Autodesk Inventor part; units mm, degrees
ref_plane "YZ Plane" through (0, 0, 0) normal (1, 0, 0) x (0, 1, 0)
ref_plane "XZ Plane" through (0, 0, 0) normal (0, 1, 0) x (-1, 0, 0)
ref_plane "XY Plane" through (0, 0, 0) normal (0, 0, 1) x (1, 0, 0)
sketch "スケッチ1" plane through (0, 0, 0) normal (0, 0, 1) x (1, 0, 0)
  line L0 (-81.3, 0) -> (81.3, 0)
  line L1 (81.3, 0) -> (81.3, 14.5)
  line L2 (81.3, 14.5) -> (-81.3, 14.5)
  line L3 (-81.3, 14.5) -> (-81.3, 0)
  line L4 (-99, 14.5) -> (99, 14.5)
  line L5 (99, 14.5) -> (99, 54.5)
  line L6 (99, 54.5) -> (-99, 54.5)
  line L7 (-99, 54.5) -> (-99, 14.5)
  point P0 (0, 0)
  point P1 (0, 0)
  point P2 (0, 14.5)
  point P3 (-81.3, 14.5)
  point P4 (81.3, 14.5)
  dimension "d0" = 162.6
  dimension "d1" = 14.5
  dimension "d2" = 198
  dimension "d3" = 40
extrude "押し出し1" add sketch "スケッチ1" along normal blind 2.5
properties part number "wall" material "木材 (カエデ材)"
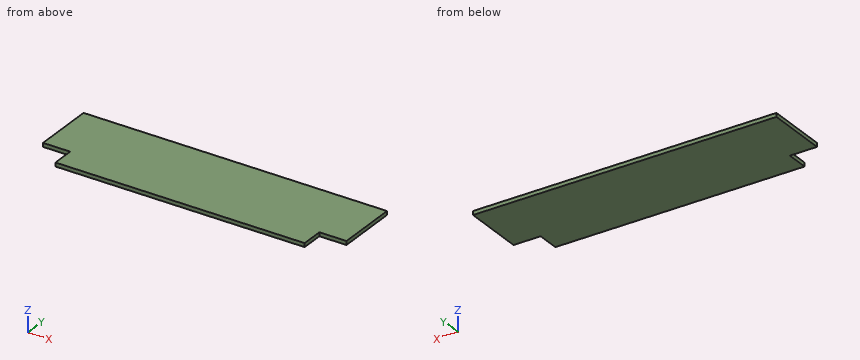
Can you work these out from the model? Positions are in its coordinate system, mm. Coordinates: 2 decimals unless noted, no trailing zeros. Write each loop counter-clockwise with the first axis right and the second up, starting at its lowest first coordinate (ties: lowest second). Pieces come first, ordered by that corner, then holes. Notation, with made-up numbers: (86, 0) -> (100, 0) arc R13 cw to (100, 21) -> close; hole circle Ø1 at (-35.5, 66). An arc over 180 degrees is marked (long way). Write each question's results on one line, items separated by ' | '. Start each with the question number.
Item 1: If we section it at A-A, the plane z = 1.4: Write out the boundary of the cut face in (x, y).
Item 2: If we section it at B-B, the plane y = 7: Write out the boundary of the cut face in (x, z).
Item 3: Please list where these lines run through material, in increasing order: probe 1 along X at (y, z) = (14, 2.4); probe 2 along Y at (x, z) = (-87.5, 0.85).
Item 4: I'm going to push flat-ended pins straight in: P1, Ø1.2, axis at y = 10, z = 1, coming from the -X side; P2, Ø0.8, axis at x = -86, z = 1, coming from the -Y side. Where does each tip first touch, or does it pass through?
Answer block:
1) outline: (-99, 14.5) -> (-81.3, 14.5) -> (-81.3, 0) -> (81.3, 0) -> (81.3, 14.5) -> (99, 14.5) -> (99, 54.5) -> (-99, 54.5) -> close
2) outline: (-81.3, 0) -> (81.3, 0) -> (81.3, 2.5) -> (-81.3, 2.5) -> close
3) probe 1: -81.3 to 81.3 | probe 2: 14.5 to 54.5
4) P1: x = -81.3 | P2: y = 14.5
